Autodesk Inventor part; units mm, degrees
ref_plane "Work Plane1" through (192, 55, 15) normal (1, 0, 0) x (0, 0, -1)
ref_plane "YZ Plane" through (0, 0, 0) normal (1, 0, 0) x (0, 1, 0)
ref_plane "XZ Plane" through (0, 0, 0) normal (0, 1, 0) x (-1, 0, 0)
sketch "Sketch1" plane through (0, 0, 0) normal (0, 0, 1) x (1, 0, 0)
  line L0 (0, 0) -> (384, 0)
  line L1 (384, 0) -> (384, 55)
  line L2 (384, 55) -> (0, 55)
  line L3 (0, 55) -> (0, 0)
  dimension "d0" = 55
  dimension "d1" = 384
extrude "Extrusion1" add sketch "Sketch1" along normal blind 15
sketch "Sketch4" plane through (0, 0, 15) normal (0, 0, 1) x (1, 0, 0)
  line L0 (0, 0) -> (15, 0)
  line L1 (15, 0) -> (15, 27.5)
  line L2 (15, 27.5) -> (0, 27.5)
  line L3 (0, 27.5) -> (0, 0)
  line L4 (384, 55) -> (0, 55)
  line L5 (192, 55) -> (192, 39.783)
  line L6 (164.5, 55) -> (219.5, 55)
  line L7 (219.5, 55) -> (219.5, 27.5)
  line L8 (219.5, 27.5) -> (164.5, 27.5)
  line L9 (164.5, 27.5) -> (164.5, 55)
  line L10 (384, 0) -> (369, 0)
  line L11 (369, 0) -> (369, 27.5)
  line L12 (369, 27.5) -> (384, 27.5)
  line L13 (384, 27.5) -> (384, 0)
  point P0 (192, 27.5)
  dimension "d23" = 15
  dimension "d24" = 27.5
  dimension "d25" = 55
extrude "Extrusion2" cut sketch "Sketch4" against normal through all
ref_plane "Work Plane1" through (192, 55, 15) normal (1, 0, 0) x (0, 0, -1)
fillet "Fillet1" radius 2 4 edges at (15, 27.5, 7.5) (164.5, 27.5, 7.5) (219.5, 27.5, 7.5) (369, 27.5, 7.5)
sketch "Sketch2" plane through (0, 55, 0) normal (0, 1, 0) x (1, 0, 0)
  line L0 (7.5, -7.5) -> (376.5, -7.5)
  line L1 (0, 0) -> (0, -15)
  line L2 (384, 0) -> (0, 0)
  point P0 (192, -7.5)
  point P1 (0, -7.5)
  point P2 (192, 0)
  dimension "d4" = 369
sketch "Sketch3" plane through (0, 0, 0) normal (0, 0, -1) x (-1, 0, 0)
  line L0 (-384, 0) -> (-384, 55)
  line L1 (0, 0) -> (-384, 0)
  line L2 (0, 55) -> (0, 0)
  line L3 (-384, 55) -> (0, 55)
  line L4 (-7.5, 10) -> (-376.5, 10)
  line L5 (-376.5, 45) -> (-7.5, 45)
  dimension "d12" = 10
  dimension "d20" = 10
  dimension "d21" = 7.5
  dimension "d22" = 7.5
equation "\"d20\" = d12"
properties part number "Breadth Board"
Input: part model. Units: mm. Frame: model coordinates. A direction names the side the tool comes from. Coordinates: 2 decimals unless noted, no trailing zeros. Order: outer loops, then holes, each group sorted by start corner. A loop starts at its lowest first (then second) coordinate and runs counter-clockwise, first axis right, second up.
1. Draft query along X for faces 1 (the flat face through (164.5, 42, 8)), 2 (the flat face through (189, 22, 15)), 3 (the flat face through (0, 41, 7)), 4 (the flat face through (219.5, 42, 8)). Return one class per face: +X half, -X half, draft (parallel to the pull), parting line (faces both ways), or undercut.
Checked values:
face 1: undercut
face 2: draft
face 3: -X half
face 4: undercut
2. Contact query for flat-ended pins moving along their axis: P1, Ø7.5, axis at y = 18.5, z = 5.5, coming from the -X side; P2, Ø4, axis at x = 7.5, z = 10, coming from the -Y side; P3, Ø8, axis at y = 15.5, z = 11, coming from the +X side. Output: stop coordinate, or through.
Checked values:
P1: stops at x = 15
P2: stops at y = 27.5
P3: stops at x = 369
3. Cut plane C-C, the plane y = 22. Return loops of the section in (x, z), plus the area to 3 significant figures.
Checked values:
outline: (15, 0) - (369, 0) - (369, 15) - (15, 15) - close
area: 5,310 mm2
4. Ray query, line 1 along X through (y, z) = (40.5, 5); line 2 along Y through (x, z) = (177, 10.75); line 3 along X through (y, z) = (5, 9.5). Return the intervals inside material, ascending.
Checked values:
line 1: x = 0 to 164.5, 219.5 to 384
line 2: y = 0 to 27.5
line 3: x = 15 to 369
5. Access query for faces 5 (the flat face through (384, 41, 7)), 6 (the flat face through (369, 13, 8)), 7 (the flat face through (303, 55, 7)), 8 (the flat face through (192, 27.5, 8)), 9 (the flat face through (15, 13, 8)). Directions: +Z, -Z, +X, -X, +Y, -Y. A direction counts if a zero-diameter tool reaches every point of the face in a straight line with its end or side. Return the directions, or none.
Checked values:
face 5: +Z, -Z, +X, +Y, -Y
face 6: +Z, -Z, +X, -Y
face 7: +Z, -Z, +X, -X, +Y
face 8: +Z, -Z, +Y
face 9: +Z, -Z, -X, -Y
6. Cut plane B-B, the plane z = 3.75. Return loops of the section in (x, y), plus the area to 3 significant figures.
Checked values:
outline: (0, 27.5) - (13, 27.5) arc R2 cw to (15, 25.5) - (15, 0) - (369, 0) - (369, 25.5) arc R2 cw to (371, 27.5) - (384, 27.5) - (384, 55) - (219.5, 55) - (219.5, 29.5) arc R2 cw to (217.5, 27.5) - (166.5, 27.5) arc R2 cw to (164.5, 29.5) - (164.5, 55) - (0, 55) - close
area: 18,800 mm2
7. Cut plane A-A, the plane y = 46.5. Return loops of the section in (x, z), plus the area to 4 significant figures.
Checked values:
outline: (0, 0) - (164.5, 0) - (164.5, 15) - (0, 15) - close; (219.5, 0) - (384, 0) - (384, 15) - (219.5, 15) - close
area: 4,935 mm2
